from build123d import *

# Parameters (mm, degrees)
SKETCH1_R           = 231.80521347
BOSS_EXTRUDE1_DEPTH = 85
SKETCH2_W           = 215.150125982
SKETCH2_H           = 209.680207524
BOSS_EXTRUDE3_DEPTH = 800
SKETCH3_R           = 35
CUT_EXTRUDE1_DEPTH  = 248
SKETCH4_R           = 150.212654375
BOSS_EXTRUDE5_DEPTH = 885


with BuildPart() as part:
    # Sketch1 → Boss-Extrude1 (new body)
    with BuildSketch(Plane.XY):
        Circle(SKETCH1_R)
    extrude(amount=BOSS_EXTRUDE1_DEPTH)

    # Sketch2 → Boss-Extrude3 (add)
    with BuildSketch(Plane.XY.offset(85)):
        Rectangle(SKETCH2_W, SKETCH2_H)
    extrude(amount=BOSS_EXTRUDE3_DEPTH)

    # Sketch3 → Cut-Extrude1 (cut)
    with BuildSketch(Plane(origin=(107.575062991, 0, 0), x_dir=(0, 0, -1), z_dir=(1, 0, 0))):
        with Locations((-795.184826294, 0)):
            Circle(SKETCH3_R)
    extrude(amount=-CUT_EXTRUDE1_DEPTH, mode=Mode.SUBTRACT)

    # Sketch4 → Boss-Extrude5 (add)
    with BuildSketch(Plane.XY.offset(885)):
        Circle(SKETCH4_R)
    extrude(amount=-BOSS_EXTRUDE5_DEPTH)


solid = part.part
Model file for the job. Use its own axes, mm. A direction names the side the tool comes from. Coordinates: 2 decimals unless noted, no trailing zeros. Order: outer loops, then holes, each group sorted by start corner. A loop starts at its lowest first (then second) coordinate and runs counter-clockwise, first axis right, second up. Notation, with made-up numbers: (-9, 51) -> (46, 51) arc R31 cw to (46, 82) -> close; hole circle Ø6 at (48.25, 36.25). An arc over 180 degrees is marked (long way). Return JSON: item names as keys, results as strings. Group by question number.
Item 1: Saw through at D-D on y = -185. Write the cut outline in (x, z).
Item 2: Saw through at C-C on z = 154. Write the cut outline in (x, y).
Item 3: Tool access for faces 1 (the cylindrical face through (-19.555, 148.934, 490.6)), 2 (the flat face through (-3, 3, 0)): list every direction of +Z, -Z, +X, -X, +Y, -Y with a clear straight run to the whole face (end or side of a thin tool).
Item 4: Flat gauge pins, fed straight in: P1, Ø1.5, axis at y = 62, z = 788.5, coming from the -X side; P2, Ø1.5, axis at x = 157, y = -141.5, coming from the -Z side; P3, Ø2, axis at x = -26.5, z = 560, coming from the +Y side; P4, Ø1.5, axis at x = 135.5, z = 669, coming from the +Y side. Where does each tip first touch, or does it go through?
Item 5: Wall check: line 1 along Z through (x, y) = (-3, -199); line 2 along X through (y, z) = (0, 262); line 3 along Y through (x, z) = (135, 196). Give the ranges that are in metal, low to high. Write a range as [from, to].
Item 6: Saw through at A-A on y = 0. Write the cut outline in (x, z).
Values found:
{
 "1": {"outline": "(-139.67, 0) -> (139.67, 0) -> (139.67, 85) -> (-139.67, 85) -> close"},
 "2": {"outline": "circle Ø300.43 at (0, 0)"},
 "3": {"face 1": "+Z", "face 2": "-Z, +X, -X, +Y, -Y"},
 "4": {"P1": "stops at x = -137.16", "P2": "stops at z = 0", "P3": "stops at y = 148.03", "P4": "stops at y = 66.38"},
 "5": {"line 1": "z = [0, 85]", "line 2": "x = [-150.21, 150.21]", "line 3": "y = [-65.87, 65.87]"},
 "6": {"outline": "(-231.81, 0) -> (231.81, 0) -> (231.81, 85) -> (150.21, 85) -> (150.21, 885) -> (-150.21, 885) -> (-150.21, 85) -> (-231.81, 85) -> close"}
}
